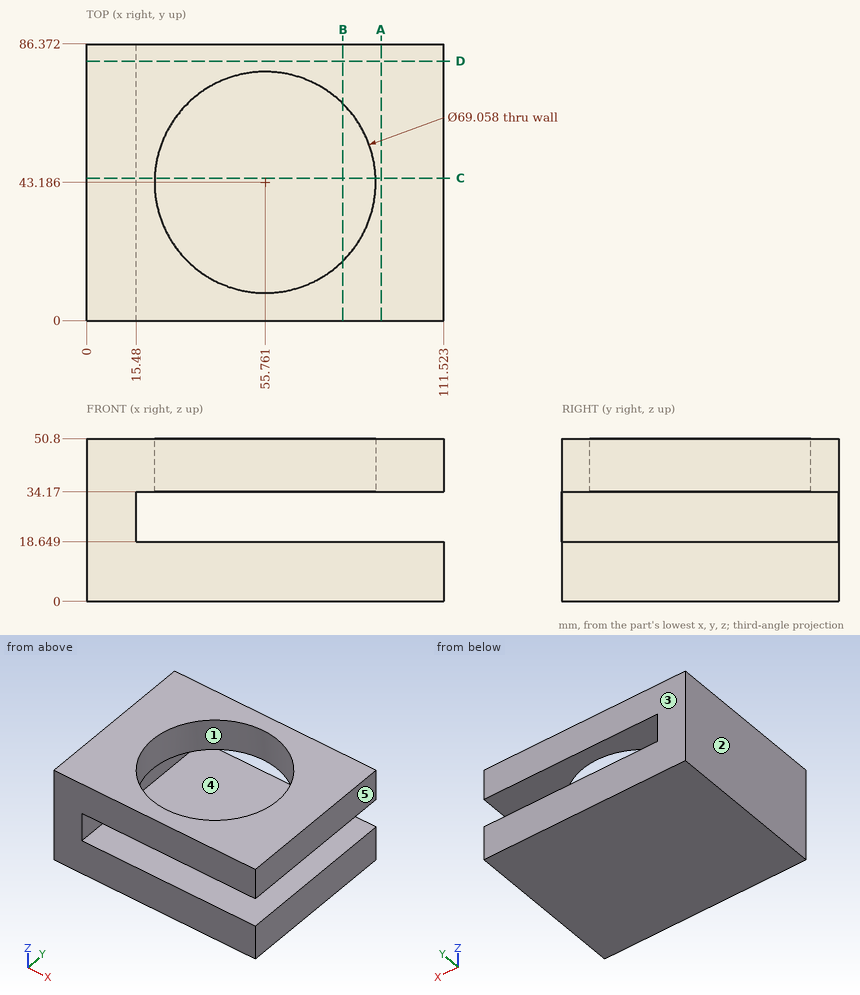
Geometry check sheet. Reference: drawing and pictorial views, mm from the part's lowest x, y, z. A direction names the side the tool comes from. Coordinates: 2 decimals unless noted, no trailing zeros. Write each loop counter-clockwise with the first axis right and the second up, starting at its lowest first coordinate (ties: lowest second). Pieces come first, ordered by that corner, then holes.
Item 1: Cross-section at D-D on y = 81. Record the boundary of the cut face in (x, z).
Numbers:
outline: (0, 0) - (111.52, 0) - (111.52, 18.65) - (15.48, 18.65) - (15.48, 34.17) - (111.52, 34.17) - (111.52, 50.8) - (0, 50.8) - close
Item 2: Depth check by flat-ended pin: pin 1 Ø1.5 at (x, z) = (45.5, 20.5) entering from -Y. Enter the tip coordinate at first touch or a pass-through.
Numbers:
pin 1: passes through
Item 3: Cross-section at A-A on x = 92. Record the boundary of the cut face in (y, z), then the cut area to 3 significant figures.
Numbers:
outline: (0, 0) - (86.37, 0) - (86.37, 18.65) - (0, 18.65) - close; (0, 34.17) - (86.37, 34.17) - (86.37, 50.8) - (0, 50.8) - close
area: 3,050 mm2
Item 4: Scan lines: probe 1 along Z at (x, y) = (107, 78); probe 2 along Z at (x, y) = (42.5, 45); probe 3 along X at (y, z) = (14, 23.5). Record each from-to range of solid material in increasing order.
Numbers:
probe 1: z = 0 to 18.65, 34.17 to 50.8
probe 2: z = 0 to 18.65
probe 3: x = 0 to 15.48
Item 5: Cross-section at C-C on y = 44.5. Record the boundary of the cut face in (x, z) (1 decimal).
Numbers:
outline: (0, 0) - (111.5, 0) - (111.5, 18.6) - (15.5, 18.6) - (15.5, 34.2) - (21.3, 34.2) - (21.3, 50.8) - (0, 50.8) - close; (90.3, 34.2) - (111.5, 34.2) - (111.5, 50.8) - (90.3, 50.8) - close
Item 6: Mould release check, pull along Y, two halves, no side actions. Record for the marked faces 1, 2 and 3: released by +Y, released by -Y, zero draft, split by the parting line, or undercut.
Numbers:
face 1: undercut
face 2: zero draft
face 3: released by +Y
Item 7: Cross-section at B-B on x = 80. Record the boundary of the cut face in (y, z) (1 decimal), then the cut area to 3 significant figures.
Numbers:
outline: (0, 0) - (86.4, 0) - (86.4, 18.6) - (0, 18.6) - close; (0, 34.2) - (18.6, 34.2) - (18.6, 50.8) - (0, 50.8) - close; (67.8, 34.2) - (86.4, 34.2) - (86.4, 50.8) - (67.8, 50.8) - close
area: 2,230 mm2
Item 8: Access from +Z, -Z, +X, -X, +Y, -Y to the whole of each face (thin tool, end or side, straight path). Record for the marked faces 4 and 5.
Numbers:
face 4: +X, +Y, -Y
face 5: +Z, -Z, +X, +Y, -Y
